from build123d import *

# Parameters (mm, degrees)
F3_DEPTH  = 18
F4_R      = 4.25
F5_DEPTH  = 30
F6_R      = 4.25
F7_DEPTH  = 100
F2_R      = 7.7
F8_DEPTH  = 24
F9_W      = 8
F9_H      = 2
F10_DEPTH = 40


with BuildPart() as f3:
    # F2 (on Front) → F3 (new body)
    with BuildSketch(Plane.XZ):
        with BuildLine():
            Line((-57.0810220509, 0), (0, 0))
            ThreePointArc((0, 0), (-2.0556624872, 6.2369382637), (-0.0810220509, 12.5))
            Line((-0.0810220509, 12.5), (-27.0810220509, 12.5))
            Line((-27.0810220509, 12.5), (-27.0810220509, 20.5))
            Line((-27.0810220509, 20.5), (-27.0810220509, 21))
            Line((-27.0810220509, 21), (-27.0810220509, 21.5))
            Line((-27.0810220509, 21.5), (-27.0810220509, 29.5))
            Line((-27.0810220509, 29.5), (-0.0810220509, 29.5))
            Line((-0.0810220509, 29.5), (0, 42))
            Line((0, 42), (-57.0810220509, 42))
            Line((-57.0810220509, 42), (-57.0810220509, 0))
        make_face()
        with BuildLine():
            ThreePointArc((-0.0810220509, 12.5), (-2.0556624872, 6.2369382637), (0, 0))
            Line((0, 0), (-0.0810220509, 12.5))
        make_face()
        Polygon((-27.0810220509, 21), (-27.0810220509, 20.5), (-0.0810220509, 20.5), (-0.0810220509, 21.5), (-27.0810220509, 21.5), align=None)
    extrude(amount=F3_DEPTH)

    # F4 (on face) → F5 (cut)
    with BuildSketch(Plane(origin=(-57.0810220509, 0, 0), x_dir=(0, -1, 0), z_dir=(-1, 0, 0))):
        with Locations((9, 6.25)):
            Circle(F4_R)
        with Locations((9, 35.75)):
            Circle(F4_R)
    extrude(amount=-F5_DEPTH, mode=Mode.SUBTRACT)

    # F6 (on face) → F7 (cut)
    with BuildSketch(Plane.XY.offset(42)):
        with Locations((-13.5, -9)):
            Circle(F6_R)
    extrude(amount=-F7_DEPTH, mode=Mode.SUBTRACT)

    # F2 (on Front) → F8 (join)
    with BuildSketch(Plane.XZ):
        with BuildLine():
            Line((-0.0810220509, 12.5), (0, 0))
            ThreePointArc((0, 0), (11.9605862967, -3.8667611144), (19.344112749, 6.3062916824))
            ThreePointArc((19.344112749, 6.3062916824), (11.894578688, 16.5006269319), (-0.0810220509, 12.5))
        make_face()
        with Locations((8.644112749, 6.3062916824)):
            Circle(F2_R, mode=Mode.SUBTRACT)
    extrude(amount=F8_DEPTH)

    # F9 (on Front) → F10 (cut)
    with BuildSketch(Plane.XZ):
        with Locations((17.9096895307, 6.058463525)):
            Rectangle(F9_W, F9_H)
    extrude(amount=F10_DEPTH, mode=Mode.SUBTRACT)


solid = f3.part
CAD build for the part. Positions are in the model's coordinates, mm. A direction names the side the tool comes from. Round coordinates to 2 decimals unless told otherwise and drop trailing zeros. Order: outer loops, then holes, each group sorted by start corner. A loop starts at its lowest first (then second) coordinate and runs counter-clockwise, first axis right, second up. Notation, with made-up numbers: (62, 25) -> (97, 25) arc R35 ccw to (97, 58) -> close; hole circle Ø1 at (57.5, 60). An arc over 180 degrees is marked (long way). Write each question's results on one line, items separated by ' | '.
1. Cut at A-A (x = -22). Give the cut face in (y, z).
Findings below:
outline: (-18, 0) -> (0, 0) -> (0, 12.5) -> (-18, 12.5) -> close; (-18, 20.5) -> (0, 20.5) -> (0, 21.5) -> (-18, 21.5) -> close; (-18, 29.5) -> (0, 29.5) -> (0, 42) -> (-18, 42) -> close
2. Cut at C-C (z = 6.25). Give the cut face in (x, y).
Findings below:
outline: (-57.08, -18) -> (-0.04, -18) -> (-0.04, -24) -> (0.94, -24) -> (0.94, 0) -> (-57.08, 0) -> (-57.08, -4.75) -> (-27.08, -4.75) -> (-27.08, -13.25) -> (-57.08, -13.25) -> close; hole circle Ø8.5 at (-13.5, -9)
3. 3-axis set-ups, long thin cutter, end or side, ignore diameter. For faces 1 (the face through (-11.54, -12.77, 35.84)), 2 (the face through (-10, -13, 21.5)), 3 (the face through (-10, -13, 12.5)), 4 (the face through (-27.081, -9, 6)), 5 (the face through (-29, -18, 21)): which of +Z, -Z, +X, -X, +Y, -Y reach the whole face in a straight line?
Findings below:
face 1: +Z, -Z | face 2: +X, +Y, -Y | face 3: +Y, -Y | face 4: -X | face 5: +Z, -Z, -X, -Y
4. Pull direction Z, two halves, no side cores. Call faces 6 (the face through (-28, -9, 42)), 7 (the face through (-11.54, -12.77, 21.01)), 8 (the face through (18, -12, 7.058)): pulls with the +Z half, pulls with the -Z half, needs draft (parallel to the pull), parting line crosses it, or undercut.
Findings below:
face 6: pulls with the +Z half | face 7: needs draft | face 8: undercut
5. Wall check: line 1 along Z through (x, y) = (-14.5, -3.75); line 2 along Z through (x, y) = (-35, -6); line 3 along Y through (x, z) = (-13.5, 21). Give the ranges that are in metal, low to high. Write a range as [from, to].
Findings below:
line 1: z = [0, 12.5], [20.5, 21.5], [29.5, 42] | line 2: z = [0, 3.24], [9.26, 32.74], [38.76, 42] | line 3: y = [-18, -13.25], [-4.75, 0]
6. Flat gauge pins, fed straight in: P1, Ø10, axis at x = 7.5, y = -18, coming from the +Z side; P2, Ø2, axis at x = -49, y = -10.5, coming from the -Z side; P3, Ø2.5, axis at y = -12.5, z = 17, coming from the +X side; P4, Ø11, axis at y = -9, z = 6.25, coming from the +X side. Where does each tip first touch, or does it go through?
Findings below:
P1: stops at z = 17.01 | P2: stops at z = 0 | P3: stops at x = 13.67 | P4: stops at x = 19.32
7. Cut at D-D (y = -15.75). Give the cut face in (x, z).
Findings below:
outline: (-57.08, 0) -> (0, 0) arc R10.7 ccw to (19.27, 5.06) -> (16.24, 5.06) arc R7.7 cw (long way) to (16.31, 7.06) -> (19.32, 7.06) arc R10.7 ccw to (-0.08, 12.5) -> (-27.08, 12.5) -> (-27.08, 20.5) -> (-0.08, 20.5) -> (-0.08, 21.5) -> (-27.08, 21.5) -> (-27.08, 29.5) -> (-0.08, 29.5) -> (0, 42) -> (-57.08, 42) -> close
8. Cut at B-B (x = -13.5). Give the cut face in (y, z), plus the area to 3 significant figures.
Findings below:
outline: (-18, 0) -> (-13.25, 0) -> (-13.25, 12.5) -> (-18, 12.5) -> close; (-18, 20.5) -> (-13.25, 20.5) -> (-13.25, 21.5) -> (-18, 21.5) -> close; (-18, 29.5) -> (-13.25, 29.5) -> (-13.25, 42) -> (-18, 42) -> close; (-4.75, 0) -> (0, 0) -> (0, 12.5) -> (-4.75, 12.5) -> close; (-4.75, 20.5) -> (0, 20.5) -> (0, 21.5) -> (-4.75, 21.5) -> close; (-4.75, 29.5) -> (0, 29.5) -> (0, 42) -> (-4.75, 42) -> close | area: 247 mm²
